Answer from the drawing. Dimensions are ordinates in mm from the lowest x, y and z of the part. A direction names the side the tool comes from. Give positions to 0.01 mm unless a question says otherwise; leave off trailing zeros. Order: outer loops, then holes, each group sorted by start corner. A loop starts at its lowest first (then second) coordinate and runs counter-clockwise, first axis right, second up. Notation, with made-up numbers: (26, 31) - (44, 31) arc R18 ccw to (44, 43) - close; hole circle Ø3 at (32, 13.5). An arc over 180 degrees is marked (long way). Write each question's results on one line, items separated by ' | '.
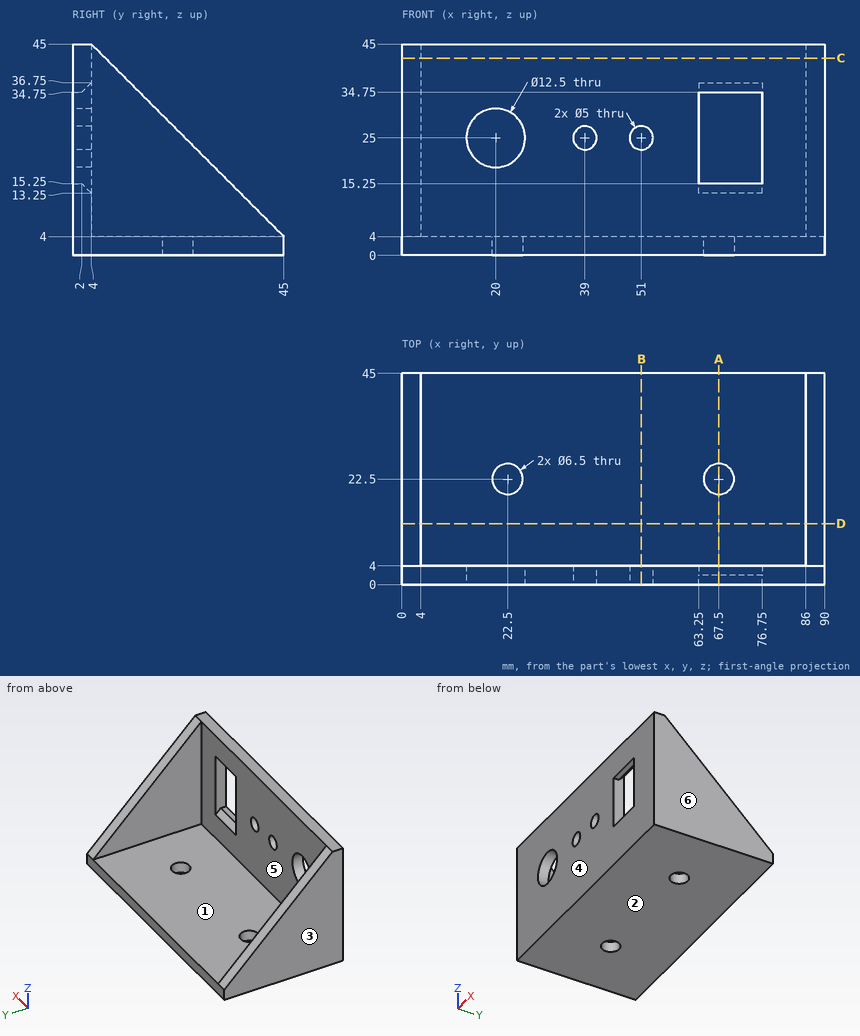
(1) Section D-D (y = 13) is taken. Give the vertices of the cut face in (x, z), plus the area to 3 significant figures.
Conclusion:
outline: (0, 0) - (90, 0) - (90, 36) - (86, 36) - (86, 4) - (4, 4) - (4, 36) - (0, 36) - close | area: 616 mm^2
(2) Consider probe 1 along X at (y, z) = (11.5, 29); probe 2 along Z at (x, y) = (20, 0.9); probe 3 along Y at (x, z) = (35.5, 29). Determine where each line is inside the solid, lowest interval first. Write a range as [from, to].
Conclusion:
probe 1: [0, 4], [86, 90] | probe 2: [0, 18.75], [31.25, 45] | probe 3: [0, 4]
(3) For the marked faces 1 and 2, determine the directions among +Z, -Z, +X, -X, +Y, -Y from which every point of the face is accessible in a straight line to the end or side of a thin tool.
Conclusion:
face 1: +Z, +Y | face 2: -Z, +X, -X, +Y, -Y
(4) Section A-A (x = 67.5) is taken. Give the vertices of the cut face in (y, z).
Conclusion:
outline: (0, 0) - (19.25, 0) - (19.25, 4) - (4, 4) - (4, 13.25) - (2, 15.25) - (0, 15.25) - close; (0, 34.75) - (2, 34.75) - (4, 36.75) - (4, 45) - (0, 45) - close; (25.75, 0) - (45, 0) - (45, 4) - (25.75, 4) - close
(5) Each of these flat-tipped pins is pushed along its axis until it touches: pin 1 (6 mm diameter, centred on x = 22.5, y = 22.5, fed in from -Z); pin 2 (4 mm diameter, centred on x = 19.5, y = 26, fed in from +Z); pin 3 (20.5 mm diameter, centred on x = 54.5, z = 32, fed in from +Y). Where does it stop, or does it pass through?
Conclusion:
pin 1: through | pin 2: z = 4 | pin 3: y = 4
(6) Section B-B (x = 51) is taken. Give the vertices of the cut face in (y, z), plus the area to 3 significant figures.
Conclusion:
outline: (0, 0) - (45, 0) - (45, 4) - (4, 4) - (4, 22.5) - (0, 22.5) - close; (0, 27.5) - (4, 27.5) - (4, 45) - (0, 45) - close | area: 324 mm^2
(7) Section C-C (z = 42) is taken. Give the vertices of the cut face in (x, y), plus the area to 3 significant figures.
Conclusion:
outline: (0, 0) - (90, 0) - (90, 7) - (86, 7) - (86, 4) - (4, 4) - (4, 7) - (0, 7) - close | area: 384 mm^2
(8) The mould has two halves that part along X. Classify the marked faces 3, 4, 5 and 6: pulls with the +X half, pulls with the -X half, needs draft (parallel to the pull), parting line crosses it, or undercut.
Conclusion:
face 3: pulls with the -X half | face 4: needs draft | face 5: undercut | face 6: pulls with the +X half
